Read the model definition and answer for the solid it produces. Units are mm, in the model's axes. Face numbers are marked on the shaded views. A direction names the side the tool comes from. Coordinates: 2 decimals unless noted, no trailing zeros. Order: outer loops, then holes, each group sorted by start corner. A loop starts at its lowest first (then second) coordinate and runs counter-clockwise, first axis right, second up. Notation, with made-up numbers: (57.5, 31) -> (98.5, 31) arc R24 ccw to (98.5, 53) -> close; hole circle Ø2 at (45.5, -32). An arc over 180 degrees is marked (long way). Return JSON: item names as keys, results as strings. Group by question number.
```python
from build123d import *

# Parameters (mm, degrees)
F1_DEPTH = 8
F3_D     = 5
F5_DEPTH = 8.001
F7_DEPTH = 12.001


with BuildPart() as f1:
    # F0 (on Top) → F1 (new body)
    with BuildSketch(Plane.XY):
        Polygon((0, 12), (0, 0), (52, 0), (60, 2.5), (60, 9.5), (52, 12), align=None)
    extrude(amount=F1_DEPTH)

    # F3 (through all)
    with Locations(Plane.XY.offset(8)):
        with Locations((6, 6)):
            Hole(F3_D / 2)

    # F4 (on face) → F5 (cut, through all)
    with BuildSketch(Plane.XY.offset(8)):
        with BuildLine():
            ThreePointArc((15, 9.0993724681), (11.825, 5.9243724681), (15, 2.7493724681))
            Line((15, 2.7493724681), (40, 2.7493724681))
            ThreePointArc((40, 2.7493724681), (43.175, 5.9243724681), (40, 9.0993724681))
            Line((40, 9.0993724681), (15, 9.0993724681))
        make_face()
    extrude(amount=-F5_DEPTH, mode=Mode.SUBTRACT)

    # F6 (on face) → F7 (cut, through all)
    with BuildSketch(Plane.XZ):
        Polygon((60, 8), (54, 8), (60, 5), align=None)
    extrude(amount=-F7_DEPTH, mode=Mode.SUBTRACT)


solid = f1.part
```
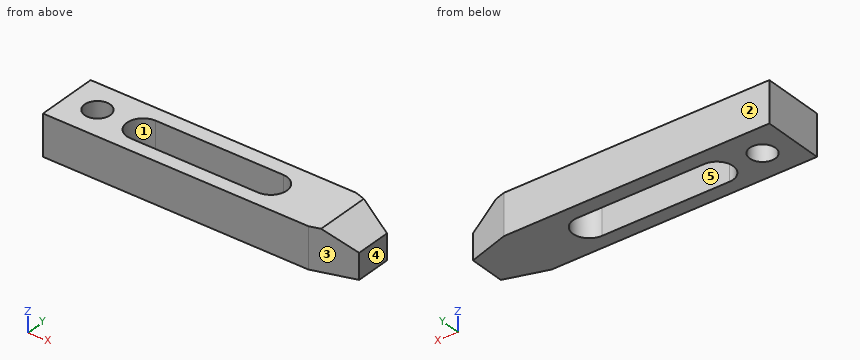
1. For a pull along X with two mould halves and no side action, classify the marked faces 1, 2 and 3 as released by +X, released by -X, zero draft, split by the parting line, or undercut.
2. Which of the six approach directions +Z, -Z, +X, -X, +Y, -Y give full straight-line access (tool end or side, diameter ignored) to the marked faces 4 and 5?
3. Given pin 1 (1.5 mm diameter, centred on x = 40.5, y = 7, fed in from -Z), flat-ended and moving along its own axis, determine where the tip first touches the part or whether it passes through.
4. Find section B-B on z = 0.5. Determine the outline of the cut face in (x, y) (3 decimals).
5. Straight lines are drawn through the part: L1, parallel to Y at x = 25, z = 2.5; L2, parallel to X at y = 5.5, z = 7.75; L3, parallel to X at y = 7.25, z = 2.5. For each, find the intervals that lie inside material, in ascending order.
6. Find section D-D on y = 6. Determine the outline of the cut face in (x, z).
7. Find section A-A on x = 34. Determine the outline of the cut face in (y, z).
8. Find section C-C on x = 6. Determine the outline of the cut face in (y, z), and give its area (3 significant figures).
Result:
{
 "1": {"face 1": "undercut", "face 2": "zero draft", "face 3": "released by +X"},
 "2": {"face 4": "+Z, -Z, +X, +Y, -Y", "face 5": "+Z, -Z"},
 "3": {"pin 1": "through"},
 "4": {"outline": "(0, 0) -> (52, 0) -> (60, 2.5) -> (60, 9.5) -> (52, 12) -> (0, 12) -> close; hole circle Ø5 at (6, 6); hole (15, 2.749) -> (40, 2.749) arc R3.175 ccw to (40, 9.099) -> (15, 9.099) arc R3.175 ccw to start"},
 "5": {"L1": "0 to 2.75, 9.1 to 12", "L2": "0 to 3.55, 8.45 to 11.85, 43.15 to 54.5", "L3": "0 to 3.83, 8.17 to 12.11, 42.89 to 60"},
 "6": {"outline": "(0, 0) -> (3.5, 0) -> (3.5, 8) -> (0, 8) -> close; (8.5, 0) -> (11.83, 0) -> (11.83, 8) -> (8.5, 8) -> close; (43.17, 0) -> (60, 0) -> (60, 5) -> (54, 8) -> (43.17, 8) -> close"},
 "7": {"outline": "(0, 0) -> (2.75, 0) -> (2.75, 8) -> (0, 8) -> close; (9.1, 0) -> (12, 0) -> (12, 8) -> (9.1, 8) -> close"},
 "8": {"outline": "(0, 0) -> (3.5, 0) -> (3.5, 8) -> (0, 8) -> close; (8.5, 0) -> (12, 0) -> (12, 8) -> (8.5, 8) -> close", "area": "56.0 mm^2"}
}
